Verification items for the finished model (mm, model axes). Face numbers are marked on the shaded views. A direction names the side the tool comes from. Give positions to 0.01 mm unless a question says otherwise; leave off trailing zeros. Write each loop counter-clockwise with the first axis right and the second up, starting at its lowest first coordinate (ties: lowest second). Pieces come first, ordered by that corner, then holes. Notation, with made-up numbers: (31.5, 66) - (52.5, 66) arc R33 cw to (52.5, 95) - close; hole circle Ø1 at (64, 37.5). An arc over 180 degrees is marked (long way). Put each result on its own line as item: value.
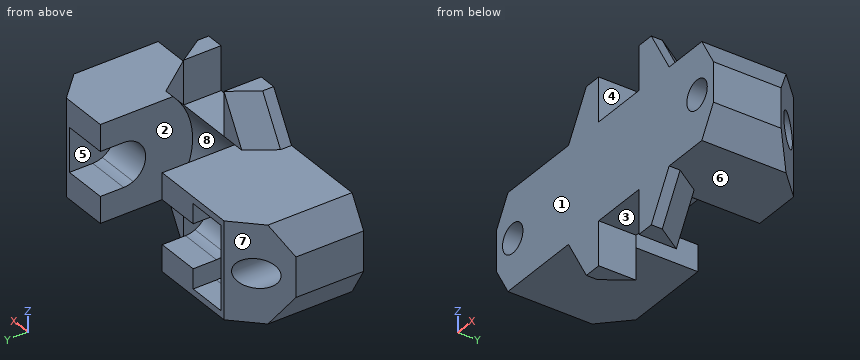
from build123d import *
from OCP.BRepFilletAPI import BRepFilletAPI_MakeChamfer

# Parameters (mm, degrees)
SKIZZE1_R                       = 1.65
AUFSATZ_LINEAR_AUSTRAGEN1_DEPTH = 12.5
SCHNITT_LINEAR_START            = -10.3
SKIZZE2_R                       = 7.85
SKIZZE2_R_2                     = 2.5
SCHNITT_LINEAR_AUSTRAGEN1_DEPTH = 10
SCHNITT_LINEAR_START_2          = -5.3
SCHNITT_LINEAR_AUSTRAGEN2_DEPTH = 20
SCHNITT_LINEAR_AUSTRAGEN3_DEPTH = 4.5
SCHNITT_LINEAR_START_3          = -11
SCHNITT_LINEAR_AUSTRAGEN4_DEPTH = 11
AUFSATZ_LINEAR_START            = -4.248884
AUFSATZ_LINEAR_AUSTRAGEN2_DEPTH = 4.248884
FASE1_SIZE                      = 3
FASE1_SIZE2                     = 1.732050808


with BuildPart() as part:
    # Skizze1 → Aufsatz-Linear austragen1 (new body)
    with BuildSketch(Plane(origin=(0, 0, 0), x_dir=(1, 0, 0), z_dir=(0, 1, 0))):
        Polygon((0, 11), (-31.34722325, 11), (-33.223611625, 7.75), (-33.223611625, 3.25), (-31.34722325, 0), (0, 0), (1.876388375, 3.25), (1.876388375, 7.75), align=None)
        with Locations(Location((-0.773611625, 5.5, 0), (0, 0, 270))):
            Circle(SKIZZE1_R, mode=Mode.SUBTRACT)
        with Locations(Location((-30.573611625, 5.5, 0), (0, 0, 270))):
            Circle(SKIZZE1_R, mode=Mode.SUBTRACT)
    extrude(amount=AUFSATZ_LINEAR_AUSTRAGEN1_DEPTH)

    # Skizze2 → Schnitt-Linear austragen1 (cut)
    with BuildSketch(Plane(origin=(1.876388375, 0, 0), x_dir=(0, 0, -1), z_dir=(1, 0, 0)).offset(SCHNITT_LINEAR_START)):
        with Locations((5.5, 9.85)):
            Circle(SKIZZE2_R)
        with Locations((5.5, 9.85)):
            Circle(SKIZZE2_R_2, mode=Mode.SUBTRACT)
    extrude(amount=-SCHNITT_LINEAR_AUSTRAGEN1_DEPTH, mode=Mode.SUBTRACT)

    # Skizze3 → Schnitt-Linear austragen2 (cut)
    with BuildSketch(Plane(origin=(1.876388375, 0, 0), x_dir=(0, 0, -1), z_dir=(1, 0, 0)).offset(SCHNITT_LINEAR_START_2)):
        with BuildLine():
            Line((7.75, 12.5), (3.25, 12.5))
            Line((3.25, 12.5), (3.25, 10.939724736))
            ThreePointArc((3.25, 10.939724736), (5.5, 12.35), (7.75, 10.939724736))
            Line((7.75, 10.939724736), (7.75, 12.5))
        make_face()
        with BuildLine():
            Line((8, 12.5), (7.75, 12.5))
            Line((7.75, 12.5), (7.75, 10.939724736))
            ThreePointArc((7.75, 10.939724736), (7.936698586, 10.409016994), (8, 9.85))
            Line((8, 9.85), (8, 12.5))
        make_face()
        with BuildLine():
            Line((3.25, 12.5), (3, 12.5))
            Line((3, 12.5), (3, 9.85))
            ThreePointArc((3, 9.85), (3.063301414, 10.409016994), (3.25, 10.939724736))
            Line((3.25, 10.939724736), (3.25, 12.5))
        make_face()
        with BuildLine():
            ThreePointArc((7.75, 10.939724736), (5.5, 12.35), (3.25, 10.939724736))
            Line((3.25, 10.939724736), (3.25, 8.760275264))
            ThreePointArc((3.25, 8.760275264), (5.5, 7.35), (7.75, 8.760275264))
            Line((7.75, 8.760275264), (7.75, 10.939724736))
        make_face()
        with BuildLine():
            ThreePointArc((3.25, 10.939724736), (3.063301414, 10.409016994), (3, 9.85))
            ThreePointArc((3, 9.85), (3.063301414, 9.290983006), (3.25, 8.760275264))
            Line((3.25, 8.760275264), (3.25, 10.939724736))
        make_face()
        with BuildLine():
            ThreePointArc((8, 9.85), (7.936698586, 10.409016994), (7.75, 10.939724736))
            Line((7.75, 10.939724736), (7.75, 8.760275264))
            ThreePointArc((7.75, 8.760275264), (7.936698586, 9.290983006), (8, 9.85))
        make_face()
    extrude(amount=-SCHNITT_LINEAR_AUSTRAGEN2_DEPTH, mode=Mode.SUBTRACT)

    # Skizze4 → Schnitt-Linear austragen3 (cut)
    with BuildSketch(Plane(origin=(-23.423611625, 0, 0), x_dir=(0, 0, -1), z_dir=(1, 0, 0))):
        with BuildLine():
            Line((10.25, 12.5), (0.75, 12.5))
            Line((0.75, 12.5), (0.75, 9.85))
            ThreePointArc((0.75, 9.85), (5.5, 5.1), (10.25, 9.85))
            Line((10.25, 9.85), (10.25, 12.5))
        make_face()
    extrude(amount=-SCHNITT_LINEAR_AUSTRAGEN3_DEPTH, mode=Mode.SUBTRACT)

    # Skizze5 → Schnitt-Linear austragen4 (cut)
    with BuildSketch(Plane.XY.offset(SCHNITT_LINEAR_START_3)):
        Polygon((1.876388375, 12.5), (-2.923611625, 12.5), (1.876388375, 7.7), align=None)
        Polygon((-33.223611625, 12.5), (-28.423611625, 12.5), (-33.223611625, 7.7), align=None)
    extrude(amount=SCHNITT_LINEAR_AUSTRAGEN4_DEPTH, mode=Mode.SUBTRACT)

    # Skizze6 → Aufsatz-Linear austragen2 (add)
    with BuildSketch(Plane.XZ.offset(AUFSATZ_LINEAR_START)):
        Polygon((-16.673611625, 0), (-16.673611625, 5), (-18.673611625, 5), (-21.560362971, 0), align=None)
        Polygon((-10.173611625, 0), (-10.173611625, 5), (-8.173611625, 5), (-5.286860279, 0), align=None)
        Polygon((-18.673611625, -16), (-21.560362971, -11), (-16.673611625, -11), (-16.673611625, -16), align=None)
        Polygon((-10.173611625, -11), (-5.286860279, -11), (-8.173611625, -16), (-10.173611625, -16), align=None)
    extrude(amount=AUFSATZ_LINEAR_AUSTRAGEN2_DEPTH)

    # Fase1: one chamfer whose edges measure the first distance from different faces: ONE call of the kernel's chamfer builder (chamfer() names one face for all edges)
    fase1_edges_1 = [part.edges().sort_by_distance(p)[0] for p in [
        (-6.730235952, 4.248884, -13.5),
    ]]
    fase1_side_1 = [part.faces().sort_by_distance(p)[0] for p in [
        (-6.730235952, 2.124442, -13.5),
    ]]
    fase1_edges_2 = [part.edges().sort_by_distance(p)[0] for p in [
        (-20.116987298, 4.248884, -13.5),
    ]]
    fase1_side_2 = [part.faces().sort_by_distance(p)[0] for p in [
        (-20.116987298, 2.124442, -13.5),
    ]]
    fase1_edges_3 = [part.edges().sort_by_distance(p)[0] for p in [
        (-6.730235952, 4.248884, 2.5),
    ]]
    fase1_side_3 = [part.faces().sort_by_distance(p)[0] for p in [
        (-6.730235952, 2.124442, 2.5),
    ]]
    fase1_edges_4 = [part.edges().sort_by_distance(p)[0] for p in [
        (-20.116987298, 4.248884, 2.5),
    ]]
    fase1_side_4 = [part.faces().sort_by_distance(p)[0] for p in [
        (-20.116987298, 2.124442, 2.5),
    ]]
    fase1 = BRepFilletAPI_MakeChamfer(part.part.solid().wrapped)
    for e in fase1_edges_1:
        fase1.Add(FASE1_SIZE, FASE1_SIZE2, e.wrapped, fase1_side_1[0].wrapped)  # the first distance lies on this face
    for e in fase1_edges_2:
        fase1.Add(FASE1_SIZE, FASE1_SIZE2, e.wrapped, fase1_side_2[0].wrapped)  # the first distance lies on this face
    for e in fase1_edges_3:
        fase1.Add(FASE1_SIZE, FASE1_SIZE2, e.wrapped, fase1_side_3[0].wrapped)  # the first distance lies on this face
    for e in fase1_edges_4:
        fase1.Add(FASE1_SIZE, FASE1_SIZE2, e.wrapped, fase1_side_4[0].wrapped)  # the first distance lies on this face
    add(Compound.cast(fase1.Shape()), mode=Mode.REPLACE)


solid = part.part
Q1. Section check C-C, the plane y = 6.5. Record the cut outline in (x, z), plus the area to 3 significant figures.
Answers follow:
outline: (-33.22, -7.75) - (-31.35, -11) - (-18.42, -11) - (-18.42, 0) - (-31.35, 0) - (-33.22, -3.25) - close; (-8.42, -11) - (0, -11) - (1.88, -7.75) - (1.88, -3.25) - (0, 0) - (-8.42, 0) - close; hole circle Ø3.3 at (-30.57, -5.5); hole (-27.92, -8.87) - (-23.42, -8.87) - (-23.42, -2.13) - (-27.92, -2.13) - close; hole circle Ø3.3 at (-0.77, -5.5)
area: 216 mm2
Q2. Section check B-B, the plane x = -25. Record the cut outline in (y, z), plus the area to 3 significant figures.
Answers follow:
outline: (0, -11) - (12.5, -11) - (12.5, -10.25) - (9.85, -10.25) arc R4.75 cw to (9.85, -0.75) - (12.5, -0.75) - (12.5, 0) - (0, 0) - close
area: 76.9 mm2
Q3. Release check for a two-part mould opening along Z. For the marked faces 5, 6, 7 and 8 record: released by +Z, released by -Z, zero draft, split by the parting line, or undercut.
Answers follow:
face 5: undercut
face 6: released by -Z
face 7: zero draft
face 8: undercut
Q4. Section check D-D, the plane z = -9.25. Record the cut outline in (x, y), plus the area to 3 significant figures.
Answers follow:
outline: (-32.36, 0) - (1.01, 0) - (1.01, 8.57) - (-2.92, 12.5) - (-8.42, 12.5) - (-8.42, 2.95) - (-18.42, 2.95) - (-18.42, 12.5) - (-23.42, 12.5) - (-23.42, 6.93) - (-27.92, 6.93) - (-27.92, 12.5) - (-28.42, 12.5) - (-32.36, 8.57) - close
area: 281 mm2
Q5. Set-up check for the marked faces 1, 2, 3 and 4: record each of +Z, -Z, +X, -X, +Y, -Y from which the full face is reachable in a straight line by a thin tool's end or side.
Answers follow:
face 1: +Z, -Z, +X, -X, -Y
face 2: +Y
face 3: -Z, +Y, -Y
face 4: +Z, +Y, -Y
Q6. Section check A-A, the plane z = -5.5. Record the cut outline in (x, y), plus the area to 3 significant figures.
Answers follow:
outline: (-33.22, 0) - (-32.22, 0) - (-32.22, 8.7) - (-33.22, 7.7) - close; (-28.92, 0) - (-2.42, 0) - (-2.42, 12) - (-2.92, 12.5) - (-3.42, 12.5) - (-3.42, 7.35) - (-8.42, 7.35) - (-8.42, 2) - (-18.42, 2) - (-18.42, 7.35) - (-23.42, 7.35) - (-23.42, 5.1) - (-27.92, 5.1) - (-27.92, 12.5) - (-28.42, 12.5) - (-28.92, 12) - close; (0.88, 0) - (1.88, 0) - (1.88, 7.7) - (0.88, 8.7) - close
area: 158 mm2
Q7. Go/stop test with flat-tipped pins: pin 1 Ø4 at (x, z) = (-30.57, -5.5) entering from +Y; pin 2 Ø4 at (x, z) = (-3.5, -7) entering from +Y; pin 3 Ø0.9 at (x, z) = (-18, -12.5) entering from +Y; pin 4 Ø1.3 at (x, y) = (-21, 11) entering from -Z. Record where each tip stops, or that it passes through.
Answers follow:
pin 1: stops at y = 12.35
pin 2: stops at y = 12.5
pin 3: stops at y = 4.25
pin 4: stops at z = -11
Q8. Scan lines: line 1 along X through (y, z) = (4.5, -5.5); line 2 along X through (y, z) = (6.5, -5.5); line 3 along Z through (x, y) = (-22, 10.5). Record each from-to range of solid material in increasing order.
Answers follow:
line 1: x = -33.22 to -32.22, -28.92 to -18.42, -8.42 to -2.42, 0.88 to 1.88
line 2: x = -33.22 to -32.22, -28.92 to -27.92, -23.42 to -18.42, -8.42 to -2.42, 0.88 to 1.88
line 3: z = -11 to -8, -3 to 0
